from build123d import *

# Parameters (mm, degrees)
CHAMFER_1_SIZE = 0.5


with BuildPart() as part:
    # 草图1 → 旋转1 (revolve)
    with BuildSketch(Plane.XY, mode=Mode.PRIVATE) as revolve_1_sk:
        Polygon((9.25, 0), (12.6, 0), (12.6, 4), (11.1, 4), (11.1, 5), (12.7, 5), (12.7, 16.5), (10.6, 16.5), (10.6, 8), (11.7, 8), (11.7, 7), (10, 7), (10, 2), (9.25, 2), align=None)
    revolve(revolve_1_sk.sketch.rotate(Axis((0, 0, 0), (0, 1, 0)), 90), axis=Axis((0, 0, 0), (0, 1, 0)))  # turned: the seam where the file's is

    # 倒角1
    chamfer_1_edges = [part.edges().sort_by_distance(p)[0] for p in [
        (0, 16.5, 10.6),
        (0, 16.5, 12.7),
        (0, 5, 12.7),
        (0, 0, 12.6),
    ]]
    chamfer(chamfer_1_edges, length=CHAMFER_1_SIZE)


solid = part.part
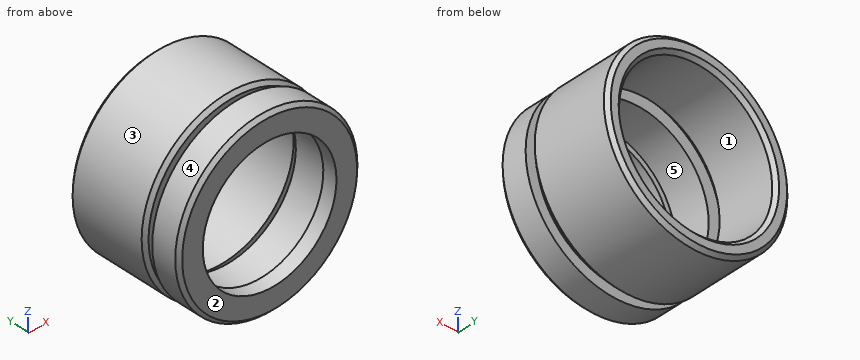
For this review, take the finished solid that the model builds, in its own axes (mm). Face numbers are marked on the shaded views. A direction names the side the tool comes from. Give positions to 0.01 mm unless a question says otherwise; leave off trailing zeros. Order: outer loops, then holes, each group sorted by start corner. A loop starts at its lowest first (then second) coordinate and runs counter-clockwise, first axis right, second up. Notation, with made-up numbers: (-28.75, 26) - (-3.75, 26) arc R10 ccw to (-3.75, 37) - close; hole circle Ø6 at (34.25, -36.5). An arc over 180 degrees is marked (long way). Answer as a JSON object with one key per item and string values. Group by question number.
Item 1: Take a section at A-A on y = 13.5. Give the boundary of the cut face in (x, z), and give its area (3 significant figures).
Item 2: Clearance check with a flat-ended pin moving along its axis: pin 1 Ø1.5 at (x, y) = (1, 4) entering from -Z. State where the tip first meets the part, or that it passes through.
Item 3: Machinability: for the marked faces 4 and 5, which of the approach directions +Z, -Z, +X, -X, +Y, -Y give a long, thin tool a straight path to every point of the face, cutting with its end or side? Answer none if there is none.
Item 4: Wall thickness on line 1 along Y through (x, z) = (11, -2.5); line 2 along X through (y, z) = (1.25, 0); line 3 along X through (y, z) = (7.7, 0): over which ranges is each line inside the solid? List them lowest first.
Item 5: Draft analysis for pull direction X (two halves, no side actions). For the marked faces 1, 2 and 3, state which applies: pulls with the +X half, pulls with the -X half, needs draft (parallel to the pull), parting line crosses it, or undercut.
Reported:
{
 "1": {"outline": "circle Ø25.4 at (0, 0); hole circle Ø21.2 at (0, 0)", "area": "154 mm^2"},
 "2": {"pin 1": "z = -12.6"},
 "3": {"face 4": "-Y", "face 5": "+Y"},
 "4": {"line 1": "0 to 4, 5 to 7, 8 to 16.5", "line 2": "-12.6 to -9.25, 9.25 to 12.6", "line 3": "-12.7 to -11.7, 11.7 to 12.7"},
 "5": {"face 1": "undercut", "face 2": "needs draft", "face 3": "parting line crosses it"}
}
